Autodesk Inventor part; units mm, degrees
ref_plane "YZ Plane" through (0, 0, 0) normal (1, 0, 0) x (0, 1, 0)
ref_plane "XZ Plane" through (0, 0, 0) normal (0, 1, 0) x (-1, 0, 0)
ref_plane "XY Plane" through (0, 0, 0) normal (0, 0, 1) x (1, 0, 0)
sketch "Sketch1" plane through (0, 0, 0) normal (0, 1, 0) x (-1, 0, 0)
  line L0 (57.15, 152.4) -> (-57.15, 152.4)
  line L1 (-57.15, 152.4) -> (-57.15, -152.4)
  line L2 (-57.15, -152.4) -> (57.15, -152.4)
  line L3 (57.15, -152.4) -> (57.15, 152.4)
  line L4 (57.15, 152.4) -> (165.1, 152.4)
  line L5 (165.1, 152.4) -> (165.1, -152.4)
  line L6 (165.1, -152.4) -> (57.15, -152.4)
  line L7 (57.15, -152.4) -> (57.15, 152.4)
  line L8 (57.15, -152.4) -> (57.15, -92.4)
  line L9 (57.15, -92.4) -> (165.1, -92.4)
  line L10 (57.15, -152.4) -> (165.1, -92.4)
  line L11 (57.15, 152.4) -> (57.15, 92.4)
  line L12 (57.15, 92.4) -> (165.1, 92.4)
  line L13 (57.15, 152.4) -> (165.1, 92.4)
  point P0 (0, 0)
  point P1 (57.15, 0)
  point P2 (0, -152.4)
  dimension "d0" = 304.8
  dimension "d1" = 114.3
  dimension "d2" = 107.95
  dimension "d3" = 60
  dimension "d4" = 60
extrude "Extrusion1" add sketch "Sketch1" along normal blind 117.5 contours L3 L2 L1 L0 | L13 L12 L3 | L12 L5 L9 L3 | L9 L10 L3
fillet "Fillet1" radius 115 1 edges at (57.15, 117.5, 0)
sketch "Sketch2" plane through (-165.1, 0, -92.4) normal (-1, 0, 0) x (0, 0, 1)
  line L0 (55.275, 83.975) -> (55.275, 72.025) construction
  line L1 (30.65, 83.975) -> (30.65, 72.025)
  line L2 (79.9, 72.025) -> (79.9, 83.975)
  arc A0 (79.9, 83.975) -> (30.65, 83.975) centre (55.275, 83.975) ccw
  arc A1 (30.65, 72.025) -> (79.9, 72.025) centre (55.275, 72.025) ccw
  line L3 (129.525, 83.975) -> (129.525, 72.025) construction
  line L4 (104.9, 83.975) -> (104.9, 72.025)
  line L5 (154.15, 72.025) -> (154.15, 83.975)
  arc A2 (154.15, 83.975) -> (104.9, 83.975) centre (129.525, 83.975) ccw
  arc A3 (104.9, 72.025) -> (154.15, 72.025) centre (129.525, 72.025) ccw
  line L6 (92.4, 0) -> (92.4, 114.666) construction
  line L7 (0, 117.5) -> (184.8, 117.5)
  line L8 (107.3, 83.975) -> (107.3, 72.025)
  arc A4 (107.3, 72.025) -> (151.75, 72.025) centre (129.525, 72.025) ccw
  line L9 (151.75, 72.025) -> (151.75, 83.975)
  arc A5 (151.75, 83.975) -> (107.3, 83.975) centre (129.525, 83.975) ccw
  line L10 (33.05, 83.975) -> (33.05, 72.025)
  arc A6 (33.05, 72.025) -> (77.5, 72.025) centre (55.275, 72.025) ccw
  line L11 (77.5, 72.025) -> (77.5, 83.975)
  arc A7 (77.5, 83.975) -> (33.05, 83.975) centre (55.275, 83.975) ccw
  point P0 (55.275, 78)
  point P1 (129.525, 78)
  point P2 (129.525, 47.4)
  point P3 (129.525, 108.6)
  point P4 (129.525, 106.2)
  point P5 (55.275, 47.4)
  point P6 (55.275, 108.6)
  dimension "d8" = 12.5
  dimension "d9" = 61.2
  dimension "d10" = 49.25
  dimension "d12" = 2.4
  dimension "d14" = 8.9
  dimension "d15" = 12.5
  dimension "d16" = 61.2
  dimension "d17" = 49.25
  dimension "d18" = 8.9
  dimension "d19" = 2.4
extrude "Extrusion2" add sketch "Sketch2" along normal blind 21.5
properties part number "Airbox"
Verification items for the finished model (mm, model axes). A direction names the side the tool comes from. Coordinates: 2 decimals unless noted, no trailing zeros. Loops run counter-clockwise (first coordinate to the right, second up) from the corner with the lowest first, then second, coordinate; pieces in that order, holes last. Notation, with made-up numbers: (84.25, 14) -> (132.25, 14) arc R27 ccw to (132.25, 46) -> close; hole circle Ø3 at (48.25, -34). An arc over 180 degrees is marked (long way). Put each result on its own line as item: value.
1. Section check A-A, the plane z = 2. Record the boundary of the cut face in (x, y).
Result set:
outline: (-165.1, 0) -> (57.15, 0) -> (57.15, 2.5) arc R115 ccw to (-57.85, 117.5) -> (-165.1, 117.5) -> close
2. Section check D-D, the plane z = -37. Record the boundary of the cut face in (x, y).
Result set:
outline: (-186.6, 47.4) -> (-165.1, 47.4) -> (-165.1, 0) -> (57.15, 0) -> (57.15, 2.5) arc R115 ccw to (-57.85, 117.5) -> (-165.1, 117.5) -> (-165.1, 108.6) -> (-186.6, 108.6) -> (-186.6, 106.2) -> (-165.1, 106.2) -> (-165.1, 49.8) -> (-186.6, 49.8) -> close
3. Thickness scan on line 1 (Y direction, x = -174, z = -19); line 2 (X direction, y = 18, z = -67); line 3 (X direction, y = 96, z = -103). Record the ranges inside material, lowest first.
Result set:
line 1: y = 55.36 to 59.16, 96.84 to 100.64
line 2: x = -165.1 to 56.1
line 3: x = -146.03 to 9.1
4. Section check C-C, the plane x = -92. Record the boundary of the cut face in (y, z), then the cut area to 3 significant figures.
Result set:
outline: (0, -133.03) -> (117.5, -133.03) -> (117.5, 133.03) -> (0, 133.03) -> close
area: 31,300 mm^2
5. Section check B-B, the plane y = 65.5. Record the boundary of the cut face in (x, z).
Result set:
outline: (-186.6, -60.87) -> (-165.1, -60.87) -> (-165.1, -92.4) -> (-57.15, -152.4) -> (38.36, -152.4) -> (38.36, 152.4) -> (-57.15, 152.4) -> (-165.1, 92.4) -> (-165.1, 60.87) -> (-186.6, 60.87) -> (-186.6, 58.37) -> (-165.1, 58.37) -> (-165.1, 15.88) -> (-186.6, 15.88) -> (-186.6, 13.38) -> (-165.1, 13.38) -> (-165.1, -13.38) -> (-186.6, -13.38) -> (-186.6, -15.88) -> (-165.1, -15.88) -> (-165.1, -58.37) -> (-186.6, -58.37) -> close
6. Mould release check, pull along Y, two halves, no side actions. Record for faces 1 (the face through (-175.7, 108.594, 36.584)), 2 (the face through (-176, 78, 14.9)), 3 (the face through (-165.1, 78, 37)), 4 (the face through (-186.6, 78, -61)): pulls with the +Y half, pulls with the -Y half, needs draft (parallel to the pull), parting line crosses it, or undercut.
Result set:
face 1: pulls with the +Y half
face 2: undercut
face 3: undercut
face 4: needs draft
7. Gauge pin test, flat ends, axial feed: P1, Ø13, axis at x = -175.5, y = 80, coming from the +Z side; P2, Ø3, axis at y = 22, z = -17.5, coming from the -X side; P3, Ø3.5, axis at x = -180, y = 77, coming from the -Z side. Record the tip position at first contact, or that the pin passes through.
Result set:
P1: stops at z = 61.75
P2: stops at x = -165.1
P3: stops at z = -61.75
8. Tool access check on faces 5 (the face through (-176, 78, 12.5)), 6 (the face through (-175.7, 106.195, -37.614)), 7 (the face through (-175.7, 47.406, -36.584)), 8 (the face through (-175.7, 108.594, -37.666)), 9 (the face through (-176, 78, -61.75)). Record the directions out of +Z, -Z, +X, -X, +Y, -Y that give a thin tool (end or side, any length) a straight path to the whole face; none if there is none.
Result set:
face 5: -X, +Y, -Y
face 6: -X
face 7: -X, -Y
face 8: -X, +Y
face 9: -Z, -X, +Y, -Y
